from build123d import *

# Parameters (mm, degrees)
F0_R     = 8.5
F1_DEPTH = 4
F2_R     = 5
F3_DEPTH = 100
F6_R     = 1.5
F7_DEPTH = 121.2


with BuildPart() as f1:
    # F0 (on Top) → F1 (new body)
    with BuildSketch(Plane.XY):
        Circle(F0_R)
    extrude(amount=F1_DEPTH)

    # F2 (on Top) → F3 (join)
    with BuildSketch(Plane.XY):
        Circle(F2_R)
    extrude(amount=F3_DEPTH)

    # F4 (on Right) → F5 (revolve)
    with BuildSketch(Plane.YZ):
        with BuildLine():
            Line((0, 104.0042367491), (0, 100))
            Line((0, 100), (5, 100))
            ThreePointArc((5, 100), (4.470554405, 102.2392282849), (2.9943426753, 104.0042367491))
            Line((2.9943426753, 104.0042367491), (0, 104.0042367491))
        make_face()
        with BuildLine():
            ThreePointArc((0, 105), (1.5777858306, 104.7445328403), (2.9943426753, 104.0042367491))
            ThreePointArc((2.9943426753, 104.0042367491), (2.1854582893, 106.243570465), (0, 107.1883887053))
            Line((0, 107.1883887053), (0, 105))
        make_face()
        with BuildLine():
            Line((0, 105), (0, 104.0042367491))
            Line((0, 104.0042367491), (2.9943426753, 104.0042367491))
            ThreePointArc((2.9943426753, 104.0042367491), (1.5777858306, 104.7445328403), (0, 105))
        make_face()
    revolve(axis=Axis((0, 0, 103.5941943526), (0, 0, -1)))

    # F6 (on face) → F7 (cut)
    with BuildSketch(Plane(origin=(0, 0, 0), x_dir=(1, 0, 0), z_dir=(0, 0, -1))):
        Circle(F6_R)
    extrude(amount=-F7_DEPTH, mode=Mode.SUBTRACT)


solid = f1.part
Geometry check sheet. Reference: the model listing, model coordinates, mm. Round coordinates to 2 decimals unless told otherwise and drop trailing zeros. Order: outer loops, then holes, each group sorted by start corner. A loop starts at its lowest first (then second) coordinate and runs counter-clockwise, first axis right, second up. Notation, with made-up numbers: M 7,-29.5 L 59,-29.5 A7 cw 59,-21.5 Z; hole C 12.5,27 d10. An arc over 180 degrees is marked long. Answer in a Markdown table with one row per item. Add a question column.
Item 1: Draft check along Y on faces 1 (the face through (2, 0, 0)), 2 (the face through (4.57, 7.167, 1.972)), 3 (the face through (-1.5, -0.07, 52.65)). Enter one of: released by +Y, released by -Y, zero draft, split by the parting line, or undercut.
Item 2: Sectioned sample at C-C, the plane y = 4. Enter the section's corners in (x, z), plus the area to 3 significant figures.
Item 3: Sectioned sample at A-A, the plane y = 0. Enter the section's corners in (x, z).
Item 4: Material ranges on L1, parallel to X at y = 0, z = 63; L2, parallel to Y at x = 1.25, z = 7.5, recorded low to high. Write a range as [from, to].
Item 5: Sectioned sample at D-D, the plane z = 31. Enter the section's corners in (x, y), plus the area to 3 significant figures.
Item 6: Depth check by flat-ended pin: pin 1 Ø1.8 at (x, y) = (0, 0) entering from -Z; pin 2 Ø3 at (y, z) = (-2.5, 70.5) entering from -X; pin 3 Ø8 at (x, z) = (-2, 11) entering from -Y; pin 4 Ø2 at (y, z) = (-5.5, 17.5) entering from -X. Enter the tip coordinate at first touch or a pass-through.
Filled in:
| question | item | result |
|---|---|---|
| 1 | face 1 | zero draft |
| 1 | face 2 | split by the parting line |
| 1 | face 3 | undercut |
| 2 | outline | M -7.5,0 L 7.5,0 L 7.5,4 L 3,4 L 3,100 A3 ccw -3,100 L -3,4 L -7.5,4 Z |
| 2 | area | 650 mm² |
| 3 | outline | M -8.5,0 L -1.5,0 L -1.5,106.79 A3 ccw -2.99,104 A5 ccw -5,100 L -5,4 L -8.5,4 Z; M 1.5,0 L 8.5,0 L 8.5,4 L 5,4 L 5,100 A5 ccw 2.99,104 A3 ccw 1.5,106.79 Z |
| 4 | L1 | x = [-5, -1.5], [1.5, 5] |
| 4 | L2 | y = [-4.84, -0.83], [0.83, 4.84] |
| 5 | outline | C 0,0 d10; hole C 0,0 d3 |
| 5 | area | 71.5 mm² |
| 6 | pin 1 | passes through |
| 6 | pin 2 | stops at x = -4.9 |
| 6 | pin 3 | stops at y = -5 |
| 6 | pin 4 | stops at x = -2.18 |
